Check sheet for the modelled part. Datum: model origin and axes. Units: mm. Face numbers are marked on the shaded views. A direction names the side the tool comes from. Round coordinates to 2 decimals unless told otherwise and drop trailing zeros. Order: outer loops, then holes, each group sorted by start corner. A loop starts at its lowest first (then second) coordinate and runs counter-clockwise, first axis right, second up.
Q1. Set-up check for the marked faces 1 and 2: record each of +Z, -Z, +X, -X, +Y, -Y from which the full face is reachable in a straight line by a thin tool's end or side.
Q2. Scan lines: probe 1 along X at (y, z) = (-3.2, 50); probe 2 along Z at (x, y) = (-0.5, 7.5); probe 3 along Y at (x, z) = (41, -52). Record each from-to range of solid material in increasing order.
Q3. Cross-section at B-B on x = 0. Record the cut outline in (y, z).
Q4. Cross-section at A-A on z = 0. Record the cut outline in (x, y).
Q5. Depth check by flat-ended pin: P1, Ø5, axis at x = -40.5, z = -24, coming from the +Y side; P2, Ø4.5, axis at x = -50, z = -30, coming from the -Y side; P3, Ø6, axis at x = -2, y = 5.5, coming from the +Z side. Enter the tip coordinate at first touch or a pass-through.
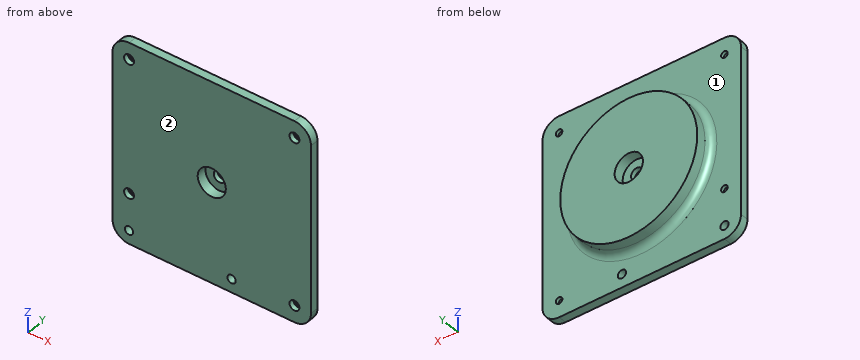
from build123d import *

# Parameters (mm, degrees)
CROQUIS1_R              = 41.4
SALIENTE_EXTRUIR1_DEPTH = 10
CROQUIS3_W              = 120
CROQUIS3_H              = 120
SALIENTE_EXTRUIR2_DEPTH = 5
CROQUIS2_R              = 3.5
CORTAR_EXTRUIR1_DEPTH   = 87.168439698
CROQUIS4_R              = 8.5
CORTAR_EXTRUIR2_DEPTH   = 6
CROQUIS5_W              = 42.3
CROQUIS5_H              = 42.3
SALIENTE_EXTRUIR3_DEPTH = 5
REDONDEO1_R             = 4
CORTAR_EXTRUIR3_REACH   = 134.292
CROQUIS8_R              = 2
CROQUIS8_R_2            = 11.5
CROQUIS9_R              = 3
CORTAR_EXTRUIR4_DEPTH   = 3
CORTAR_EXTRUIR5_REACH   = 98.188
CROQUIS10_R             = 2
CROQUIS11_W             = 17
CROQUIS11_H             = 42.3
SALIENTE_EXTRUIR4_DEPTH = 3
CROQUIS12_W             = 17
CROQUIS12_H             = 42.3
SALIENTE_EXTRUIR5_DEPTH = 3
CROQUIS15_W             = 17
CROQUIS15_H             = 3
SALIENTE_EXTRUIR6_DEPTH = 14
CROQUIS16_W             = 17
CROQUIS16_H             = 3
SALIENTE_EXTRUIR7_DEPTH = 15
CROQUIS13_R             = 2.5
CORTAR_EXTRUIR6_DEPTH   = 10
CROQUIS17_W             = 139.545471549
CROQUIS17_H             = 43.797559685
CORTAR_EXTRUIR7_DEPTH   = 120
REDONDEO2_R             = 10
REDONDEO3_R             = 10
REDONDEO4_R             = 10
REDONDEO5_R             = 10
CROQUIS18_R             = 8.55
CORTAR_EXTRUIR8_DEPTH   = 6.2


with BuildPart() as part:
    # Croquis1 → Saliente-Extruir1 (new body)
    with BuildSketch(Plane(origin=(0, 0, 0), x_dir=(1, 0, 0), z_dir=(0, 1, 0))):
        with Locations(Location((0, 0, 0), (0, 0, 270))):
            Circle(CROQUIS1_R)
    extrude(amount=SALIENTE_EXTRUIR1_DEPTH)

    # Croquis3 → Saliente-Extruir2 (add)
    with BuildSketch(Plane.XZ):
        Rectangle(CROQUIS3_W, CROQUIS3_H)
    extrude(amount=SALIENTE_EXTRUIR2_DEPTH)

    # Croquis2 → Cortar-Extruir1 (cut, through all)
    with BuildSketch(Plane(origin=(0, 10, 0), x_dir=(1, 0, 0), z_dir=(0, 1, 0))):
        with Locations(Location((0, 0, 0), (0, 0, 270))):
            Circle(CROQUIS2_R)
    extrude(amount=-CORTAR_EXTRUIR1_DEPTH, mode=Mode.SUBTRACT)

    # Croquis4 → Cortar-Extruir2 (cut)
    with BuildSketch(Plane.XZ.offset(5)):
        with Locations(Location((0, 0, 0), (0, 0, 270))):
            Circle(CROQUIS4_R)
    extrude(amount=-CORTAR_EXTRUIR2_DEPTH, mode=Mode.SUBTRACT)

    # Croquis5 → Saliente-Extruir3 (add)
    with BuildSketch(Plane.XY.offset(-43)):
        with Locations((-19.5, -26.15)):
            Rectangle(CROQUIS5_W, CROQUIS5_H)
    extrude(amount=-SALIENTE_EXTRUIR3_DEPTH)

    # Redondeo1
    redondeo1_edges = [part.edges().sort_by_distance(p)[0] for p in [
        (0, 0, -41.4),
    ]]
    fillet(redondeo1_edges, radius=REDONDEO1_R)

    # Croquis8 → Cortar-Extruir3 (cut, up to next)
    with BuildSketch(Plane(origin=(0, 0, -48), x_dir=(-1, 0, 0), z_dir=(0, 0, -1)), mode=Mode.PRIVATE) as cortar_extruir3_sk1:
        with Locations((4, -10.65)):
            Circle(CROQUIS8_R)
    cortar_extruir3_tool1 = extrude(cortar_extruir3_sk1.sketch, amount=-CORTAR_EXTRUIR3_REACH, mode=Mode.PRIVATE) & part.part
    # Croquis8 → Cortar-Extruir3 (cut, up to next)
    with BuildSketch(Plane(origin=(0, 0, -48), x_dir=(-1, 0, 0), z_dir=(0, 0, -1)), mode=Mode.PRIVATE) as cortar_extruir3_sk2:
        with Locations((35, -10.65)):
            Circle(CROQUIS8_R)
    cortar_extruir3_tool2 = extrude(cortar_extruir3_sk2.sketch, amount=-CORTAR_EXTRUIR3_REACH, mode=Mode.PRIVATE) & part.part
    # Croquis8 → Cortar-Extruir3 (cut, up to next)
    with BuildSketch(Plane(origin=(0, 0, -48), x_dir=(-1, 0, 0), z_dir=(0, 0, -1)), mode=Mode.PRIVATE) as cortar_extruir3_sk3:
        with Locations((35, -41.65)):
            Circle(CROQUIS8_R)
    cortar_extruir3_tool3 = extrude(cortar_extruir3_sk3.sketch, amount=-CORTAR_EXTRUIR3_REACH, mode=Mode.PRIVATE) & part.part
    # Croquis8 → Cortar-Extruir3 (cut, up to next)
    with BuildSketch(Plane(origin=(0, 0, -48), x_dir=(-1, 0, 0), z_dir=(0, 0, -1)), mode=Mode.PRIVATE) as cortar_extruir3_sk4:
        with Locations((4, -41.65)):
            Circle(CROQUIS8_R)
    cortar_extruir3_tool4 = extrude(cortar_extruir3_sk4.sketch, amount=-CORTAR_EXTRUIR3_REACH, mode=Mode.PRIVATE) & part.part
    # Croquis8 → Cortar-Extruir3 (cut, up to next)
    with BuildSketch(Plane(origin=(0, 0, -48), x_dir=(-1, 0, 0), z_dir=(0, 0, -1)), mode=Mode.PRIVATE) as cortar_extruir3_sk5:
        with Locations((19.5, -26.15)):
            Circle(CROQUIS8_R_2)
    cortar_extruir3_tool5 = extrude(cortar_extruir3_sk5.sketch, amount=-CORTAR_EXTRUIR3_REACH, mode=Mode.PRIVATE) & part.part
    add(cortar_extruir3_tool1.solids().sort_by_distance((-4, -10.65, -48))[0], mode=Mode.SUBTRACT)
    add(cortar_extruir3_tool2.solids().sort_by_distance((-35, -10.65, -48))[0], mode=Mode.SUBTRACT)
    add(cortar_extruir3_tool3.solids().sort_by_distance((-35, -41.65, -48))[0], mode=Mode.SUBTRACT)
    add(cortar_extruir3_tool4.solids().sort_by_distance((-4, -41.65, -48))[0], mode=Mode.SUBTRACT)
    add(cortar_extruir3_tool5.solids().sort_by_distance((-19.5, -26.15, -48))[0], mode=Mode.SUBTRACT)

    # Croquis9 → Cortar-Extruir4 (cut)
    with BuildSketch(Plane.XZ.offset(5)):
        with Locations(Location((-50, 50, 0), (0, 0, 270))):
            Circle(CROQUIS9_R)
        with Locations(Location((50, 50, 0), (0, 0, 270))):
            Circle(CROQUIS9_R)
        with Locations(Location((50, -50, 0), (0, 0, 270))):
            Circle(CROQUIS9_R)
        with Locations(Location((-50, -30, 0), (0, 0, 270))):
            Circle(CROQUIS9_R)
    extrude(amount=-CORTAR_EXTRUIR4_DEPTH, mode=Mode.SUBTRACT)

    # Croquis10 → Cortar-Extruir5 (cut, up to next)
    with BuildSketch(Plane.XZ.offset(2), mode=Mode.PRIVATE) as cortar_extruir5_sk1:
        with Locations(Location((-50, 50, 0), (0, 0, 270))):
            Circle(CROQUIS10_R)
    cortar_extruir5_tool1 = extrude(cortar_extruir5_sk1.sketch, amount=-CORTAR_EXTRUIR5_REACH, mode=Mode.PRIVATE) & part.part
    # Croquis10 → Cortar-Extruir5 (cut, up to next)
    with BuildSketch(Plane.XZ.offset(2), mode=Mode.PRIVATE) as cortar_extruir5_sk2:
        with Locations(Location((50, 50, 0), (0, 0, 270))):
            Circle(CROQUIS10_R)
    cortar_extruir5_tool2 = extrude(cortar_extruir5_sk2.sketch, amount=-CORTAR_EXTRUIR5_REACH, mode=Mode.PRIVATE) & part.part
    # Croquis10 → Cortar-Extruir5 (cut, up to next)
    with BuildSketch(Plane.XZ.offset(2), mode=Mode.PRIVATE) as cortar_extruir5_sk3:
        with Locations(Location((50, -50, 0), (0, 0, 270))):
            Circle(CROQUIS10_R)
    cortar_extruir5_tool3 = extrude(cortar_extruir5_sk3.sketch, amount=-CORTAR_EXTRUIR5_REACH, mode=Mode.PRIVATE) & part.part
    # Croquis10 → Cortar-Extruir5 (cut, up to next)
    with BuildSketch(Plane.XZ.offset(2), mode=Mode.PRIVATE) as cortar_extruir5_sk4:
        with Locations(Location((-50, -30, 0), (0, 0, 270))):
            Circle(CROQUIS10_R)
    cortar_extruir5_tool4 = extrude(cortar_extruir5_sk4.sketch, amount=-CORTAR_EXTRUIR5_REACH, mode=Mode.PRIVATE) & part.part
    add(cortar_extruir5_tool1.solids().sort_by_distance((-50, -2, 50))[0], mode=Mode.SUBTRACT)
    add(cortar_extruir5_tool2.solids().sort_by_distance((50, -2, 50))[0], mode=Mode.SUBTRACT)
    add(cortar_extruir5_tool3.solids().sort_by_distance((50, -2, -50))[0], mode=Mode.SUBTRACT)
    add(cortar_extruir5_tool4.solids().sort_by_distance((-50, -2, -30))[0], mode=Mode.SUBTRACT)

    # Croquis11 → Saliente-Extruir4 (add)
    with BuildSketch(Plane(origin=(1.65, 0, 0), x_dir=(0, 0, -1), z_dir=(1, 0, 0))):
        with Locations((51.5, -26.15)):
            Rectangle(CROQUIS11_W, CROQUIS11_H)
    extrude(amount=SALIENTE_EXTRUIR4_DEPTH)

    # Croquis12 → Saliente-Extruir5 (add)
    with BuildSketch(Plane.ZY.offset(40.65)):
        with Locations((-51.5, -26.15)):
            Rectangle(CROQUIS12_W, CROQUIS12_H)
    extrude(amount=SALIENTE_EXTRUIR5_DEPTH)

    # Croquis15 → Saliente-Extruir6 (add)
    with BuildSketch(Plane.ZY.offset(43.65)):
        with Locations((-51.5, -6.5)):
            Rectangle(CROQUIS15_W, CROQUIS15_H)
    extrude(amount=SALIENTE_EXTRUIR6_DEPTH)

    # Croquis16 → Saliente-Extruir7 (add)
    with BuildSketch(Plane(origin=(4.65, 0, 0), x_dir=(0, 0, -1), z_dir=(1, 0, 0))):
        with Locations((51.5, -6.5)):
            Rectangle(CROQUIS16_W, CROQUIS16_H)
    extrude(amount=SALIENTE_EXTRUIR7_DEPTH)

    # Croquis13 → Cortar-Extruir6 (cut)
    with BuildSketch(Plane(origin=(0, 0, 0), x_dir=(1, 0, 0), z_dir=(0, 1, 0))):
        with Locations(Location((-50, 52, 0), (0, 0, 270))):
            Circle(CROQUIS13_R)
        with Locations(Location((12, 52, 0), (0, 0, 270))):
            Circle(CROQUIS13_R)
    extrude(amount=-CORTAR_EXTRUIR6_DEPTH, mode=Mode.SUBTRACT)

    # Croquis17 → Cortar-Extruir7 (cut)
    with BuildSketch(Plane(origin=(0, 0, -60), x_dir=(-1, 0, 0), z_dir=(0, 0, -1))):
        with Locations((9.772735774, -26.898779843)):
            Rectangle(CROQUIS17_W, CROQUIS17_H)
    extrude(amount=-CORTAR_EXTRUIR7_DEPTH, mode=Mode.SUBTRACT)

    # Redondeo2
    redondeo2_edges = [part.edges().sort_by_distance(p)[0] for p in [
        (60, -2.5, -60),
    ]]
    fillet(redondeo2_edges, radius=REDONDEO2_R)

    # Redondeo3
    redondeo3_edges = [part.edges().sort_by_distance(p)[0] for p in [
        (-60, -2.5, -60),
    ]]
    fillet(redondeo3_edges, radius=REDONDEO3_R)

    # Redondeo4
    redondeo4_edges = [part.edges().sort_by_distance(p)[0] for p in [
        (-60, -2.5, 60),
    ]]
    fillet(redondeo4_edges, radius=REDONDEO4_R)

    # Redondeo5
    redondeo5_edges = [part.edges().sort_by_distance(p)[0] for p in [
        (60, -2.5, 60),
    ]]
    fillet(redondeo5_edges, radius=REDONDEO5_R)

    # Croquis18 → Cortar-Extruir8 (cut)
    with BuildSketch(Plane(origin=(0, 10, 0), x_dir=(1, 0, 0), z_dir=(0, 1, 0))):
        with Locations(Location((0, 0, 0), (0, 0, 270))):
            Circle(CROQUIS18_R)
    extrude(amount=-CORTAR_EXTRUIR8_DEPTH, mode=Mode.SUBTRACT)


solid = part.part
Results found:
1. face 1: +Y
1. face 2: +Z, -Z, +X, -X, -Y
2. probe 1: x = -60 to -53, -47 to 47, 53 to 60
2. probe 2: z = -41.4 to -8.54, 8.54 to 41.4
2. probe 3: y = -5 to 0
3. outline: (-5, -60) - (0, -60) - (0, -45.4) arc R4 cw to (4, -41.4) - (10, -41.4) - (10, -8.55) - (3.8, -8.55) - (3.8, -3.5) - (1, -3.5) - (1, -8.5) - (-5, -8.5) - close; (-5, 8.5) - (1, 8.5) - (1, 3.5) - (3.8, 3.5) - (3.8, 8.55) - (10, 8.55) - (10, 41.4) - (4, 41.4) arc R4 cw to (0, 45.4) - (0, 60) - (-5, 60) - close
4. outline: (-60, -5) - (-8.5, -5) - (-8.5, 1) - (-3.5, 1) - (-3.5, 3.8) - (-8.55, 3.8) - (-8.55, 10) - (-41.4, 10) - (-41.4, 4) arc R4 cw to (-45.4, 0) - (-60, 0) - close; (3.5, 1) - (8.5, 1) - (8.5, -5) - (60, -5) - (60, 0) - (45.4, 0) arc R4 cw to (41.4, 4) - (41.4, 10) - (8.55, 10) - (8.55, 3.8) - (3.5, 3.8) - close
5. P1: stops at y = 0.09
5. P2: stops at y = -2
5. P3: stops at z = 41.65
